from build123d import *

# Parameters (mm, degrees)
SKETCH1_R           = 1.75
SKETCH1_R_2         = 1.45
SKETCH1_R_3         = 8.25
BOSS_EXTRUDE1_DEPTH = 3
FILLET1_R           = 5


with BuildPart() as part:
    # Sketch1 → Boss-Extrude1 (new body)
    with BuildSketch(Plane(origin=(0, 0, 0), x_dir=(1, 0, 0), z_dir=(0, 1, 0))):
        with BuildLine():
            Line((54.2, 54.2), (0, 54.2))
            Line((0, 54.2), (-24.601445865, 28.330976799))
            ThreePointArc((-24.601445865, 28.330976799), (-27.87353462, 16.063982402), (-19.326300343, 6.676197648))
            Line((-19.326300343, 6.676197648), (0, 0))
            Line((0, 0), (54.2, 0))
            Line((54.2, 0), (54.2, 54.2))
        make_face()
        with Locations((5, 5)):
            Circle(SKETCH1_R, mode=Mode.SUBTRACT)
        with Locations((17.9, 3.6)):
            Circle(SKETCH1_R_2, mode=Mode.SUBTRACT)
        with Locations((49.2, 5)):
            Circle(SKETCH1_R, mode=Mode.SUBTRACT)
        with Locations((5, 49.2)):
            Circle(SKETCH1_R, mode=Mode.SUBTRACT)
        with Locations((50.4, 27.1)):
            Circle(SKETCH1_R_2, mode=Mode.SUBTRACT)
        with Locations((17.9, 50.6)):
            Circle(SKETCH1_R_2, mode=Mode.SUBTRACT)
        with Locations((49.2, 49.2)):
            Circle(SKETCH1_R, mode=Mode.SUBTRACT)
        with Locations((-15, 19.2)):
            Circle(SKETCH1_R_3, mode=Mode.SUBTRACT)
    extrude(amount=BOSS_EXTRUDE1_DEPTH)

    # Fillet1
    fillet1_edges = [part.edges().sort_by_distance(p)[0] for p in [
        (0, 1.5, 0),
        (0, 1.5, -54.2),
        (54.2, 1.5, -54.2),
        (54.2, 1.5, 0),
    ]]
    fillet(fillet1_edges, radius=FILLET1_R)


solid = part.part
Can you work these out from the model? Positions are in its coordinate system, mm. Round coordinates to 2 decimals unless told otherwise and drop trailing zeros. Write each loop counter-clockwise with the first axis right and the second up, starting at its lowest first coordinate (ties: lowest second). Pieces come first, ordered by that corner, then holes. Notation, with made-up numbers: (78, 63.25) -> (91, 63.25) arc R10 cw to (91, 80.25) -> close; hole circle Ø11 at (4, 30). An arc over 180 degrees is marked (long way). Use one line per item in the form item = value. Start each with the question number.
Q1. If I drill on probe 1 along Z at (x, y) = (17.9, 1.4); probe 2 along Z at (x, y) = (5, 1.5); probe 3 along X at (y, z) = (1.95, -49), over which ranges is the centre line in solid material (lowest first)? Write a range as [from, to].
Q2. We'd pull the mould along X, two halves only. Please class faces 1 (the face through (51.739, 1.479, -26.545)), 2 (the face through (0.2, 1.521, -53.806)), 3 (the face through (22, 0, -27)): +X half, -X half, draft (parallel to the pull), parting line (faces both ways), or undercut.
Q3. Imagine slicing it at C-C (x = -15). Please give me the cut outline in (y, z).
Q4. Imagine slicing it at D-D (z = -38). Please give me the cut outline in (x, y).
Q5. Imagine slicing it at A-A (x = 17.9). Please give me the cut outline in (y, z), then the cut area to 3 significant figures.
Q6. Imagine slicing it at B-B (y = 2.5). Count the separate pieces of the cut face and the enclosed holes in it, then the cut area to 3 significant figures.
Worked out:
q1.probe_1 = [-54.2, -52.05], [-49.15, -5.05], [-2.15, 0]
q1.probe_2 = [-54.2, -50.95], [-47.45, -6.75], [-3.25, 0]
q1.probe_3 = [-4.95, 3.26], [6.74, 47.46], [50.94, 54.2]
q2.face_1 = undercut
q2.face_2 = -X half
q2.face_3 = draft
q3.outline = (0, -38.43) -> (3, -38.43) -> (3, -27.45) -> (0, -27.45) -> close; (0, -10.95) -> (3, -10.95) -> (3, -5.18) -> (0, -5.18) -> close
q4.outline = (-15.41, 0) -> (54.2, 0) -> (54.2, 3) -> (-15.41, 3) -> close
q5.outline = (0, -54.2) -> (3, -54.2) -> (3, -52.05) -> (0, -52.05) -> close; (0, -49.15) -> (3, -49.15) -> (3, -5.05) -> (0, -5.05) -> close; (0, -2.15) -> (3, -2.15) -> (3, 0) -> (0, 0) -> close
q5.area = 145 mm^2
q6.separate_pieces = 1
q6.enclosed_holes = 8
q6.area = 3,610 mm^2
